```python
from build123d import *

# Parameters (mm, degrees)
BOSS_EXTRUDE1_DEPTH                                 = 1.2
SKETCH2_R                                           = 3.115
BOSS_EXTRUDE2_DEPTH                                 = 5.27
SKETCH3_R                                           = 5.7
BOSS_EXTRUDE3_DEPTH                                 = 2.65
CUT_EXTRUDE1_DEPTH                                  = 3.65
CUT_EXTRUDE2_DEPTH                                  = 3.65
CUT_EXTRUDE3_DEPTH                                  = 3.65
CUT_EXTRUDE4_DEPTH                                  = 3.65
CUT_EXTRUDE5_DEPTH                                  = 3.65
CUT_EXTRUDE6_DEPTH                                  = 3.65
CUT_EXTRUDE7_DEPTH                                  = 3.65
CUT_EXTRUDE8_DEPTH                                  = 3.65
CBORE_FOR_2_BINDING_HEAD_MACHINE_SCREW1_D           = 2.43
CBORE_FOR_2_BINDING_HEAD_MACHINE_SCREW1_DEPTH       = 19.12
CBORE_FOR_2_BINDING_HEAD_MACHINE_SCREW1_CBORE_D     = 4.2
CBORE_FOR_2_BINDING_HEAD_MACHINE_SCREW1_CBORE_DEPTH = 7.5
CHAMFER1_SIZE                                       = 0.6
CHAMFER1_SIZE2                                      = 2.5
SCALE1_SCALE                                        = 0.65


with BuildPart() as part:
    # Sketch1 → Boss-Extrude1 (new body)
    with BuildSketch(Plane.XY.offset(19.12)):
        with BuildLine():
            Line((-3.275, 2.296600749), (-3.275, -2.296600749))
            ThreePointArc((-3.275, -2.296600749), (0, -4), (3.275, -2.296600749))
            Line((3.275, -2.296600749), (3.275, 2.296600749))
            ThreePointArc((3.275, 2.296600749), (0, 4), (-3.275, 2.296600749))
        make_face()
    extrude(amount=-BOSS_EXTRUDE1_DEPTH)

    # Sketch2 → Boss-Extrude2 (add)
    with BuildSketch(Plane(origin=(0, 0, 17.92), x_dir=(-1, 0, 0), z_dir=(0, 0, -1))):
        Circle(SKETCH2_R)
    extrude(amount=BOSS_EXTRUDE2_DEPTH)

    # Sketch3 → Boss-Extrude3 (add)
    with BuildSketch(Plane.XY.offset(12.65)):
        Circle(SKETCH3_R)
    extrude(amount=-BOSS_EXTRUDE3_DEPTH)

    # Sketch4 → Cut-Extrude1 (cut, through all)
    with BuildSketch(Plane.XY.offset(12.65)):
        with BuildLine():
            ThreePointArc((-5.220198487, 2.289001477), (-5.670846635, 0.575759012), (-5.573734722, -1.193097334))
            ThreePointArc((-5.573734722, -1.193097334), (-5.173403948, 0.525253836), (-5.220198487, 2.289001477))
        make_face()
    extrude(amount=-CUT_EXTRUDE1_DEPTH, mode=Mode.SUBTRACT)

    # Sketch5 → Cut-Extrude2 (cut, through all)
    with BuildSketch(Plane.XY.offset(12.65)):
        with BuildLine():
            ThreePointArc((-2.072669282, 5.309806215), (-3.602771009, 4.417017213), (-4.784872834, 3.097578403))
            ThreePointArc((-4.784872834, 3.097578403), (-3.286738464, 4.029559562), (-2.072669282, 5.309806215))
        make_face()
    extrude(amount=-CUT_EXTRUDE2_DEPTH, mode=Mode.SUBTRACT)

    # Sketch6 → Cut-Extrude3 (cut, through all)
    with BuildSketch(Plane.XY.offset(12.65)):
        with BuildLine():
            ThreePointArc((2.289001477, 5.220198487), (0.575759012, 5.670846635), (-1.193097334, 5.573734722))
            ThreePointArc((-1.193097334, 5.573734722), (0.525253836, 5.173403948), (2.289001477, 5.220198487))
        make_face()
    extrude(amount=-CUT_EXTRUDE3_DEPTH, mode=Mode.SUBTRACT)

    # Sketch7 → Cut-Extrude4 (cut, through all)
    with BuildSketch(Plane.XY.offset(12.65)):
        with BuildLine():
            ThreePointArc((5.309806215, 2.072669282), (4.417017213, 3.602771009), (3.097578403, 4.784872834))
            ThreePointArc((3.097578403, 4.784872834), (4.029559562, 3.286738464), (5.309806215, 2.072669282))
        make_face()
    extrude(amount=-CUT_EXTRUDE4_DEPTH, mode=Mode.SUBTRACT)

    # Sketch8 → Cut-Extrude5 (cut, through all)
    with BuildSketch(Plane.XY.offset(12.65)):
        with BuildLine():
            ThreePointArc((5.220198487, -2.289001477), (5.670846635, -0.575759012), (5.573734722, 1.193097334))
            ThreePointArc((5.573734722, 1.193097334), (5.173403948, -0.525253836), (5.220198487, -2.289001477))
        make_face()
    extrude(amount=-CUT_EXTRUDE5_DEPTH, mode=Mode.SUBTRACT)

    # Sketch9 → Cut-Extrude6 (cut, through all)
    with BuildSketch(Plane.XY.offset(12.65)):
        with BuildLine():
            ThreePointArc((2.072669282, -5.309806215), (3.602771009, -4.417017213), (4.784872834, -3.097578403))
            ThreePointArc((4.784872834, -3.097578403), (3.286738464, -4.029559562), (2.072669282, -5.309806215))
        make_face()
    extrude(amount=-CUT_EXTRUDE6_DEPTH, mode=Mode.SUBTRACT)

    # Sketch10 → Cut-Extrude7 (cut, through all)
    with BuildSketch(Plane.XY.offset(12.65)):
        with BuildLine():
            ThreePointArc((-2.289001477, -5.220198487), (-0.575759012, -5.670846635), (1.193097334, -5.573734722))
            ThreePointArc((1.193097334, -5.573734722), (-0.525253836, -5.173403948), (-2.289001477, -5.220198487))
        make_face()
    extrude(amount=-CUT_EXTRUDE7_DEPTH, mode=Mode.SUBTRACT)

    # Sketch11 → Cut-Extrude8 (cut, through all)
    with BuildSketch(Plane.XY.offset(12.65)):
        with BuildLine():
            ThreePointArc((-5.309806215, -2.072669282), (-4.417017213, -3.602771009), (-3.097578403, -4.784872834))
            ThreePointArc((-3.097578403, -4.784872834), (-4.029559562, -3.286738464), (-5.309806215, -2.072669282))
        make_face()
    extrude(amount=-CUT_EXTRUDE8_DEPTH, mode=Mode.SUBTRACT)

    # Sketch12 → Revolve1 (revolve)
    with BuildSketch(Plane.XZ):
        Polygon((1.75, 10), (0, 10), (0, 0), (1.75, 0), (2.4, 4.8), (1.75, 4.8), align=None)
    revolve(axis=Axis((0, 0, 10), (0, 0, -1)))

    # CBORE for #2 Binding Head Machine Screw1
    with Locations(Plane.XY.offset(19.12)):
        with Locations((0, 0)):
            CounterBoreHole(CBORE_FOR_2_BINDING_HEAD_MACHINE_SCREW1_D / 2, CBORE_FOR_2_BINDING_HEAD_MACHINE_SCREW1_CBORE_D / 2, CBORE_FOR_2_BINDING_HEAD_MACHINE_SCREW1_CBORE_DEPTH, depth=CBORE_FOR_2_BINDING_HEAD_MACHINE_SCREW1_DEPTH)

    # Chamfer1
    chamfer1_edges = [part.edges().sort_by_distance(p)[0] for p in [
        (-1.75, 0, 10),
    ]]
    chamfer1_side = [part.faces().sort_by_distance(p)[0] for p in [
        (-5.016561239, 0.509329652, 10),
    ]]
    chamfer(chamfer1_edges, length=CHAMFER1_SIZE, length2=CHAMFER1_SIZE2, reference=chamfer1_side[0])


with BuildPart() as part_1:
    # Scale1: scaled about (0, 0, 11.614719244)
    add(part.part.scale(SCALE1_SCALE).moved(Location((0, 0, 4.065151735))))


solid = part_1.part
```
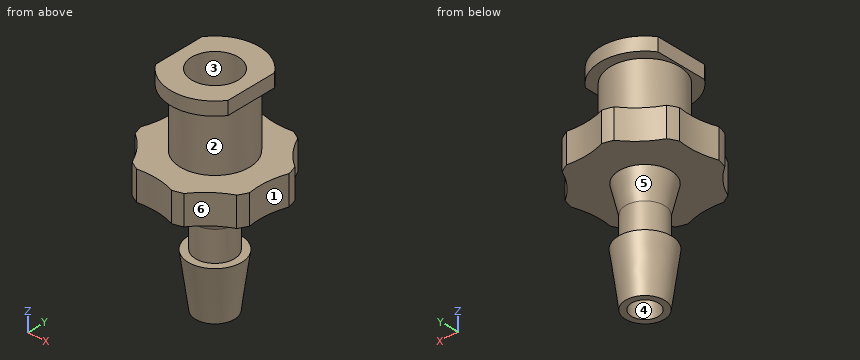
Read the model definition and answer for the solid it produces. Units are mm, in the model's axes. Face numbers are marked on the shaded views. A direction names the side the tool comes from. Give positions to 0.01 mm unless a question says otherwise; leave off trailing zeros. Order: outer loops, then holes, each group sorted by start corner. A loop starts at its lowest first (then second) coordinate and runs counter-clockwise, first axis right, second up. Notation, with made-up numbers: (87.5, -2.5) -> (118.5, -2.5) arc R9 ccw to (118.5, 7.5) -> close; hole circle Ø11 at (24.5, -36.75). An arc over 180 degrees is marked (long way). Write item = value, one per line.
1. A cutting plane is placed at B-B, the plane z = 12.5. Write down the section's boundary in (x, y) (1 decimal).
Numbers:
outline = circle Ø4 at (0, 0); hole circle Ø2.7 at (0, 0)
2. Given pin 1 (4 mm diameter, centred on y = -0.5, z = 7.5, fed in from +X); pin 2 (2 mm diameter, centred on x = 2, y = 3, fed in from -Z), each flat-ended and moving along its own axis, determine where each tip first touches the part or whether it passes through.
Numbers:
pin_1 = 1.56
pin_2 = 10.57
3. For the marked faces 1, 2 and 3, determine the directions among +Z, -Z, +X, -X, +Y, -Y from which every point of the face is accessible in a straight line to the end or side of a thin tool.
Numbers:
face_1 = +Z, -Z, +X
face_2 = none
face_3 = +Z
4. Straight lines are drawn through the part: line 1 along Y through (x, z) = (0, 15.3) (3 decimals); line 2 along Z through (x, y) = (0, -2.5); line 3 along Z through (x, y) = (2.5, -1). For each, find the intervals that lie inside material, in ascending order.
Numbers:
line_1 = -2.025 to -1.365, 1.365 to 2.025
line_2 = 10.57 to 12.29, 15.71 to 16.49
line_3 = 10.57 to 12.29
5. The mould has two halves that part along X. Classify the marked faces 4, 5 and 6: +X half, -X half, draft (parallel to the pull), parting line (faces both ways), or undercut.
Numbers:
face_4 = undercut
face_5 = parting line
face_6 = +X half
6. A cutting plane is placed at D-D, the plane z = 8.5. Write down the section's boundary in (x, y) (1 decimal).
Numbers:
outline = circle Ø2.3 at (0, 0); hole circle Ø1.6 at (0, 0)
